Autodesk Inventor part; units mm, degrees
ref_plane "YZ Plane" through (0, 0, 0) normal (1, 0, 0) x (0, 1, 0)
ref_plane "XZ Plane" through (0, 0, 0) normal (0, 1, 0) x (-1, 0, 0)
ref_plane "XY Plane" through (0, 0, 0) normal (0, 0, 1) x (1, 0, 0)
sketch "スケッチ1" plane through (0, 0, 0) normal (0, 0, 1) x (1, 0, 0)
  circle A0 centre (0, 0) radius 3.5
  dimension "d0" = 7
extrude "押し出し1" add sketch "スケッチ1" along normal blind 0.7
sketch "スケッチ2" plane through (0, 0, 0) normal (0, 0, -1) x (-1, 0, 0)
  circle A0 centre (0, 0) radius 1.5
  dimension "d3" = 3
extrude "押し出し2" add sketch "スケッチ2" along normal blind 6
thread "ねじ1"
fillet "フィレット1" radius 0.7 1 edges at (-3.5, 0, 0.7)
properties part number "ネジ低頭m3.06" material "鋼、高強度、低合金"
The listing builds one solid part. Answer for the finished solid, in the listing's coordinates (mm). A direction names the side the tool comes from. Give positions to 0.01 mm unless a question says otherwise; leave off trailing zeros. Order: outer loops, then holes, each group sorted by start corner. A loop starts at its lowest first (then second) coordinate and runs counter-clockwise, first axis right, second up. Notation, with made-up numbers: (47, 59.5) -> (79, 59.5) arc R34 cw to (79, 97.5) -> close; hole circle Ø5 at (-19, 51.5). An arc over 180 degrees is marked (long way). Answer as a JSON object with one key per item and string values. Group by question number.
Item 1: Flat-ended cylindrical pins translate along their axes: pin 1 (2 mm diameter, centred on y = -1.5, z = -2, fed in from +X); pin 2 (1.5 mm diameter, centred on x = 2, z = -4, fed in from +Y). Find the tip coordinate at first contact, or state that the pin passes through.
Item 2: The part is cut by section C-C on z = -0.5. Write down the section's boundary in (x, y).
Item 3: Consider L1, parallel to Z at x = 2.5, y = 0.75; L2, parallel to Y at x = 0, z = -1.25; L3, parallel to X at y = 1, z = -2.25. Determine where each line is inside the solid, lowest interval first. Write a range as from..to.
Item 4: A tool of negligible diameter and unlimited length cuts with its end or side. For faces 1 (the flat face through (0, 0, 0.7)), 2 (the cylindrical face through (1.5, -0.07, -2.96)), from which of +Z, -Z, +X, -X, +Y, -Y can it reach the whole face along a straight path? Write none if from no direction.
Result set:
{
 "1": {"pin 1": "x = 1.41", "pin 2": "y = 0.83"},
 "2": {"outline": "circle Ø3 at (0, 0)"},
 "3": {"L1": "0..0.7", "L2": "-1.5..1.5", "L3": "-1.12..1.12"},
 "4": {"face 1": "+Z, +X, -X, +Y, -Y", "face 2": "-Z"}
}
